from build123d import *

# Parameters (mm, degrees)
BOSS_EXTRUDE1_DEPTH = 224
SKETCH2_R           = 1.25
CUT_EXTRUDE1_DEPTH  = 225


with BuildPart() as part:
    # Sketch1 → Boss-Extrude1 (new body)
    with BuildSketch(Plane(origin=(0, 0, 0), x_dir=(1, 0, 0), z_dir=(0, 1, 0))):
        Polygon((0, 5.75), (0, 0), (5.75, 0), (5.75, 2), (9.25, 2), (9.25, 0), (15, 0), (15, 5.75), (13, 5.75), (13, 9.25), (15, 9.25), (15, 15), (9.25, 15), (9.25, 13), (5.75, 13), (5.75, 15), (0, 15), (0, 9.25), (2, 9.25), (2, 5.75), align=None)
    extrude(amount=BOSS_EXTRUDE1_DEPTH)

    # Sketch2 → Cut-Extrude1 (cut, through all)
    with BuildSketch(Plane(origin=(0, 224, 0), x_dir=(1, 0, 0), z_dir=(0, 1, 0))):
        with Locations((7.5, 7.5)):
            Circle(SKETCH2_R)
    extrude(amount=-CUT_EXTRUDE1_DEPTH, mode=Mode.SUBTRACT)


solid = part.part
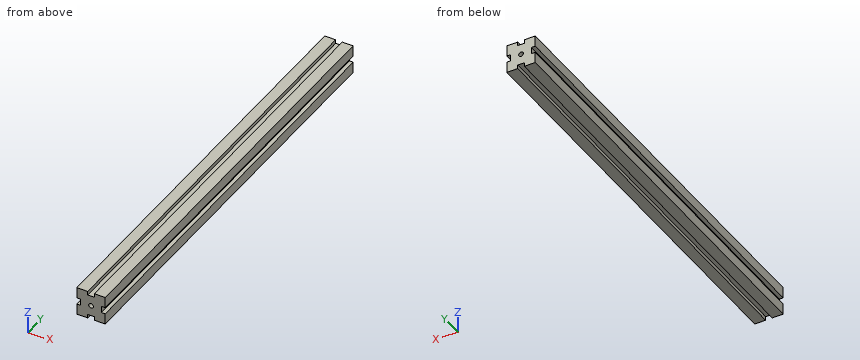
For this review, take the finished solid that the model builds, in its own axes (mm). Round coordinates to 2 decimals unless told otherwise and drop trailing zeros. Write each loop counter-clockwise with the first axis right and the second up, starting at its lowest first coordinate (ties: lowest second). Pieces come first, ordered by that corner, then holes. Notation, with made-up numbers: (-22, -5.75) -> (-9, -5.75) arc R20 ccw to (-9, 13.25) -> close; hole circle Ø1 at (15, 12). An arc over 180 degrees is marked (long way). Use CSV: the item, a comma, the result in double quotes.
(1) Clearance check with a flat-ended pin moving along its axis: P1, Ø2, axis at x = 7.5, z = -7.5, coming from the +Y side. State where the tip first meets the part, or that it passes through.
Computed values:
P1,"through"
(2) Consider section A-A, the plane y = 155. Give the boundary of the cut face in (x, z), plus the area to 3 significant figures.
Computed values:
outline,"(0, -15) -> (5.75, -15) -> (5.75, -13) -> (9.25, -13) -> (9.25, -15) -> (15, -15) -> (15, -9.25) -> (13, -9.25) -> (13, -5.75) -> (15, -5.75) -> (15, 0) -> (9.25, 0) -> (9.25, -2) -> (5.75, -2) -> (5.75, 0) -> (0, 0) -> (0, -5.75) -> (2, -5.75) -> (2, -9.25) -> (0, -9.25) -> close; hole circle Ø2.5 at (7.5, -7.5)"
area,"192 mm²"
(3) To check wall thickness, follow L1, parallel to Z at x = 7.5, y = 78; L2, parallel to X at y = 71, z = -7.75; L3, parallel to X at y = 205.5, z = -1. State the ranges of each line that lie inside material, in increasing order. Write a range as [from, to].
Computed values:
L1,"[-13, -8.75], [-6.25, -2]"
L2,"[2, 6.28], [8.72, 13]"
L3,"[0, 5.75], [9.25, 15]"
